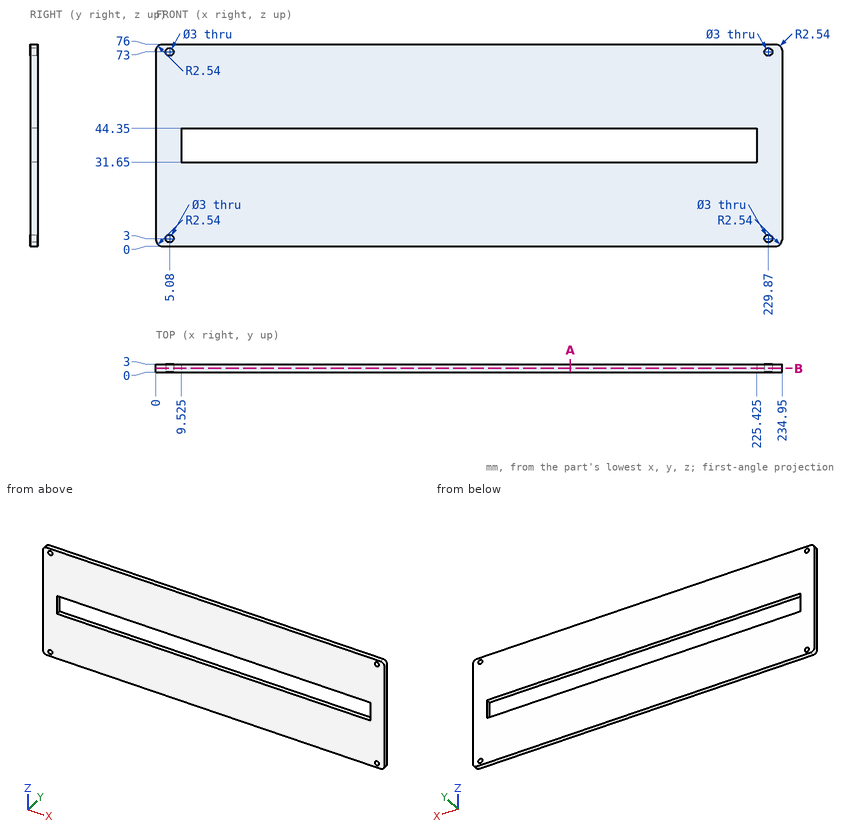
The figure shows three views and two pictorial views of one solid part (mm, origin at its lowest corner). Answer the questions. Coordinates: 2 decimals unless noted, no trailing zeros. Write each loop counter-clockwise with the first axis right and the second up, starting at its lowest first coordinate (ties: lowest second). Pieces come first, ordered by that corner, then holes.
1. Consider line 1 along X through (y, z) = (2.2, 3); line 2 along Z through (x, y) = (229.87, 0.6); line 3 along Z through (x, y) = (160.5, 1.95). Determine where each line is inside the solid, lowest interval first.
Results list:
line 1: x = 0 to 3.58, 6.58 to 228.37, 231.37 to 234.95
line 2: z = 0 to 1.5, 4.5 to 71.5, 74.5 to 76
line 3: z = 0 to 31.65, 44.35 to 76
2. The part is cut by section A-A, the plane x = 155.5. Write down the section's boundary in (y, z), and give its area (3 significant figures).
Results list:
outline: (0, 0) - (3, 0) - (3, 31.65) - (0, 31.65) - close; (0, 44.35) - (3, 44.35) - (3, 76) - (0, 76) - close
area: 190 mm2
3. The part is cut by section B-B, the plane y = 1.5. Write down the section's boundary in (x, z) (3 decimals).
Results list:
outline: (0, 2.54) arc R2.54 ccw to (2.54, 0) - (232.41, 0) arc R2.54 ccw to (234.95, 2.54) - (234.95, 73.46) arc R2.54 ccw to (232.41, 76) - (2.54, 76) arc R2.54 ccw to (0, 73.46) - close; hole circle Ø3 at (5.08, 3); hole circle Ø3 at (5.08, 73); hole (9.525, 31.65) - (225.425, 31.65) - (225.425, 44.35) - (9.525, 44.35) - close; hole circle Ø3 at (229.87, 3); hole circle Ø3 at (229.87, 73)
